```python
from build123d import *

# Parameters (mm, degrees)
SKETCH1_W            = 100
SKETCH1_H            = 90
SKETCH1_R            = 4.2
SKETCH1_R_2          = 8.125
SKETCH1_W_2          = 29.6
SKETCH1_H_2          = 22.35
SKETCH1_W_3          = 12.1
SKETCH1_H_3          = 19.35
BOSS_EXTRUDE1_DEPTH  = 3
M3_CLEARANCE_HOLE1_D = 3.6
MIRROR2_COPY_1_D     = 3.6
CHAMFER1_SIZE        = 1.5


with BuildPart() as part:
    # Sketch1 → Boss-Extrude1 (new body)
    with BuildSketch(Plane.XY):
        Rectangle(SKETCH1_W, SKETCH1_H)
        with Locations((25, 25)):
            Circle(SKETCH1_R, mode=Mode.SUBTRACT)
        with Locations((-25, 25)):
            Circle(SKETCH1_R, mode=Mode.SUBTRACT)
        with Locations((-25, -5)):
            Circle(SKETCH1_R_2, mode=Mode.SUBTRACT)
        with Locations((0, -27.825)):
            Rectangle(SKETCH1_W_2, SKETCH1_H_2, mode=Mode.SUBTRACT)
        with Locations((25, -5)):
            Rectangle(SKETCH1_W_3, SKETCH1_H_3, mode=Mode.SUBTRACT)
    extrude(amount=BOSS_EXTRUDE1_DEPTH)

    # M3 Clearance Hole1 (through all)
    with Locations(Plane.XY.offset(3)):
        with Locations((-45.5, 40.5)):
            m3_clearance_hole1 = Hole(M3_CLEARANCE_HOLE1_D / 2)

    # Mirror1: M3 Clearance Hole1 across plane
    add(m3_clearance_hole1.mirror(Plane.ZX), mode=Mode.SUBTRACT)

    # Mirror2: M3 Clearance Hole1 across plane
    add(m3_clearance_hole1.mirror(Plane(origin=(0, 0, 0), x_dir=(0, 0, 1), z_dir=(1, 0, 0))), mode=Mode.SUBTRACT)

    # Mirror2 copy 1 (through all)
    with Locations(Plane(origin=(0, 0, 3), x_dir=(-1, 0, 0), z_dir=(0, 0, 1))):
        with Locations((-45.5, 40.5)):
            Hole(MIRROR2_COPY_1_D / 2)

    # Chamfer1
    chamfer1_edges = [part.edges().sort_by_distance(p)[0] for p in [
        (25, 4.675, 3),
        (25, -14.675, 3),
    ]]
    chamfer(chamfer1_edges, length=CHAMFER1_SIZE)


solid = part.part
```
Could you check a few things on this model? Use its own coordinates, in mm. A direction names the side the tool comes from. Coordinates: 2 decimals unless noted, no trailing zeros. Loops run counter-clockwise (first coordinate to the right, second up) from the corner with the lowest first, then second, coordinate; pieces in that order, holes last.
1) Imagine slicing it at D-D (y = -40.5). List the corners of the cut face in (x, z) for me, and give its area (3 significant figures).
Reported:
outline: (-50, 0) - (-47.3, 0) - (-47.3, 3) - (-50, 3) - close; (-43.7, 0) - (43.7, 0) - (43.7, 3) - (-43.7, 3) - close; (47.3, 0) - (50, 0) - (50, 3) - (47.3, 3) - close
area: 278 mm2
2) Will these pins go through, and if not, where does the flat tip stop? pin 1 Ø6 at (x, y) = (-45.5, -40.5) entering from +Z; pin 2 Ø1.5 at (x, y) = (-8.5, -18.5) entering from +Z.
Reported:
pin 1: stops at z = 3
pin 2: passes through
3) Imagine slicing it at C-C (y = -27). List the corners of the cut face in (x, z) for me, and give its area (3 significant figures).
Reported:
outline: (-50, 0) - (-14.8, 0) - (-14.8, 3) - (-50, 3) - close; (14.8, 0) - (50, 0) - (50, 3) - (14.8, 3) - close
area: 211 mm2
4) Imagine slicing it at B-B (x = 25). List the corners of the cut face in (y, z) for me (3 decimals), and give its area (4 significant figures).
Reported:
outline: (-45, 0) - (-14.675, 0) - (-14.675, 1.5) - (-16.175, 3) - (-45, 3) - close; (4.675, 0) - (20.8, 0) - (20.8, 3) - (6.175, 3) - (4.675, 1.5) - close; (29.2, 0) - (45, 0) - (45, 3) - (29.2, 3) - close
area: 184.5 mm2
5) Please list where these lines run through material, in increasing order: line 1 along Y through (x, z) = (-25, 0.75) (3 decimals); line 2 along Y through (x, z) = (45.5, 2.15); line 3 along X through (y, z) = (23.5, 0.2).
Reported:
line 1: y = -45 to -13.125, 3.125 to 20.8, 29.2 to 45
line 2: y = -45 to -42.3, -38.7 to 38.7, 42.3 to 45
line 3: x = -50 to -28.92, -21.08 to 21.08, 28.92 to 50
6) Imagine slicing it at A-A (y = -5). List the corners of the cut face in (x, z) for me (3 decimals).
Reported:
outline: (-50, 0) - (-33.125, 0) - (-33.125, 3) - (-50, 3) - close; (-16.875, 0) - (18.95, 0) - (18.95, 3) - (-16.875, 3) - close; (31.05, 0) - (50, 0) - (50, 3) - (31.05, 3) - close
7) Thinking about a two-plate mould opening in X: for faces 1 (the face through (-1, 1, 0)), 2 (the face through (50, -1, 1)), 3 (the face through (14.8, -28, 1)), which applies, released by +X, released by -X, zero draft, split by the parting line, or undercut?
Reported:
face 1: zero draft
face 2: released by +X
face 3: undercut
8) Which directions (+Z, -Z, +X, -X, +Y, -Y) give clear straight access to the entire face, cutting with the end or side of a thin tool? Please do faces 4 (the face through (-1, 1, 3)), 5 (the face through (-14.8, -28, 1)).
Reported:
face 4: +Z, +X, -X, +Y, -Y
face 5: +Z, -Z
